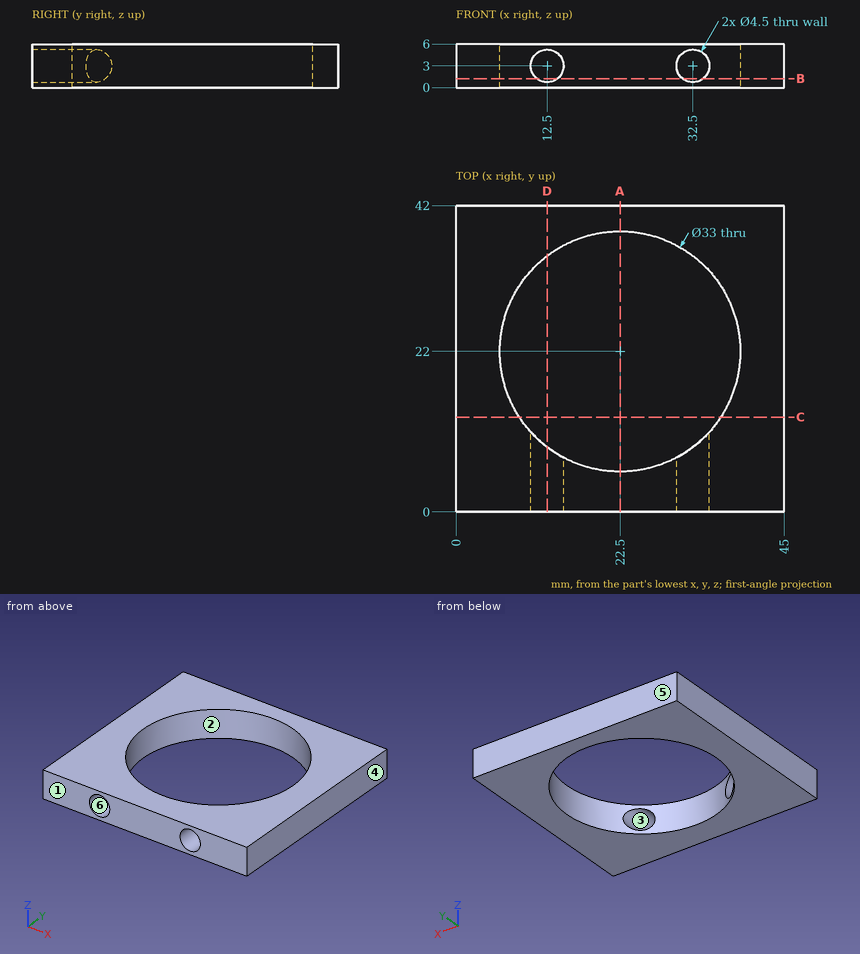
The figure shows three views and two pictorial views of one solid part (mm, origin at its lowest corner). Answer the questions. A direction names the side the tool comes from. Round coordinates to 2 decimals unless told otherwise and drop trailing zeros. Order: outer loops, then holes, each group sorted by start corner. A loop starts at its lowest first (then second) coordinate and runs counter-clockwise, first axis right, second up. Notation, with made-up numbers: (87, -12) - (144, -12) arc R21 cw to (144, 21) - close; hole circle Ø5 at (53.5, -18.75). An arc over 180 degrees is marked (long way). Write item = value, one per line. Start each with the question number.
1) For the marked faces 5 and 6, determine the directions among +Z, -Z, +X, -X, +Y, -Y from which every point of the face is accessible in a straight line to the end or side of a thin tool.
2) Section A-A, the plane x = 22.5 is taken. Write down the section's boundary in (y, z), plus the area to 3 significant figures.
3) Straight lines are drawn through the part: L1, parallel to Y at x = 22.5, z = 2; L2, parallel to X at y = 3, z = 3; L3, parallel to X at y = 7.25, z = 3. For each, find the intervals that lie inside material, in ascending order.
4) For a pull along X with two mould halves and no side action, classify the marked faces 1, 2, 3 and 4 as released by +X, released by -X, zero draft, split by the parting line, or undercut.
5) Section C-C, the plane y = 13 is taken. Write down the section's boundary in (x, z), plus the area to 3 significant figures.
6) Section D-D, the plane x = 12.5 is taken. Write down the section's boundary in (y, z), plus the area to 3 significant figures.
7) Section B-B, the plane z = 1.25 is taken. Write down the section's boundary in (x, y), plus the area to 3 significant figures.
Results list:
q1.face_5 = +Z, -Z, +X, -X, +Y
q1.face_6 = -Y
q2.outline = (0, 0) - (5.5, 0) - (5.5, 6) - (0, 6) - close; (38.5, 0) - (42, 0) - (42, 6) - (38.5, 6) - close
q2.area = 54.0 mm^2
q3.L1 = 0 to 5.5, 38.5 to 42
q3.L2 = 0 to 10.25, 14.75 to 30.25, 34.75 to 45
q3.L3 = 0 to 10.25, 14.75 to 15.1, 29.9 to 30.25, 34.75 to 45
q4.face_1 = zero draft
q4.face_2 = undercut
q4.face_3 = undercut
q4.face_4 = released by +X
q5.outline = (0, 0) - (8.67, 0) - (8.67, 6) - (0, 6) - close; (36.33, 0) - (45, 0) - (45, 6) - (36.33, 6) - close
q5.area = 104 mm^2
q6.outline = (0, 0) - (8.88, 0) - (8.88, 0.75) - (0, 0.75) - close; (0, 5.25) - (8.88, 5.25) - (8.88, 6) - (0, 6) - close; (35.12, 0) - (42, 0) - (42, 6) - (35.12, 6) - close
q6.area = 54.6 mm^2
q7.outline = (0, 0) - (11.09, 0) - (11.09, 10.09) arc R16.5 cw (long way) to (33.91, 10.09) - (33.91, 0) - (45, 0) - (45, 42) - (0, 42) - close; (13.91, 0) - (31.09, 0) - (31.09, 7.91) arc R16.5 cw to (13.91, 7.91) - close
q7.area = 984 mm^2
